```python
from build123d import *

# Parameters (mm, degrees)
F0_R     = 1.5
F1_DEPTH = 50
F2_R     = 12
F3_R     = 5
F5_DEPTH = 4
F6_SIZE  = 2.5


with BuildPart() as f1:
    # F0 (on Top) → F1 (new body)
    with BuildSketch(Plane.XY):
        with BuildLine():
            Line((40.1261364576, -50), (50, -50))
            Line((50, -50), (50, -40.1261364576))
            ThreePointArc((50, -40.1261364576), (48.5323223277, -39.658202653), (47, -39.5))
            Line((47, -39.5), (47, -47))
            Line((47, -47), (39.5, -47))
            ThreePointArc((39.5, -47), (39.658202653, -48.5323223277), (40.1261364576, -50))
        make_face()
        with BuildLine():
            Line((-40.1261364576, -50), (40.1261364576, -50))
            ThreePointArc((40.1261364576, -50), (39.658202653, -48.5323223277), (39.5, -47))
            Line((39.5, -47), (-39.5, -47))
            ThreePointArc((-39.5, -47), (-39.658202653, -48.5323223277), (-40.1261364576, -50))
        make_face()
        with BuildLine():
            ThreePointArc((47, -39.5), (48.5323223277, -39.658202653), (50, -40.1261364576))
            Line((50, -40.1261364576), (50, 40.1261364576))
            ThreePointArc((50, 40.1261364576), (48.5323223277, 39.658202653), (47, 39.5))
            Line((47, 39.5), (47, -39.5))
        make_face()
        with BuildLine():
            Line((-50, -50), (-40.1261364576, -50))
            ThreePointArc((-40.1261364576, -50), (-39.658202653, -48.5323223277), (-39.5, -47))
            Line((-39.5, -47), (-44, -47))
            Line((-44, -47), (-47, -47))
            ThreePointArc((-47, -47), (-50.0530276117, -44.8189291928), (-52.9544285232, -42.4398705103))
            ThreePointArc((-52.9544285232, -42.4398705103), (-53.9803824114, -44.2569612852), (-54.4659740059, -46.2863949669))
            ThreePointArc((-54.4659740059, -46.2863949669), (-52.2760251532, -48.1949550771), (-50, -50))
        make_face()
        with BuildLine():
            ThreePointArc((47, -39.5), (41.6966991411, -41.6966991411), (39.5, -47))
            Line((39.5, -47), (47, -47))
            Line((47, -47), (47, -39.5))
        make_face()
        with Locations((44, -44)):
            Circle(F0_R, mode=Mode.SUBTRACT)
        with BuildLine():
            ThreePointArc((47, 39.5), (48.5323223277, 39.658202653), (50, 40.1261364576))
            Line((50, 40.1261364576), (50, 50))
            Line((50, 50), (40.1261364576, 50))
            ThreePointArc((40.1261364576, 50), (39.658202653, 48.5323223277), (39.5, 47))
            Line((39.5, 47), (44, 47))
            Line((44, 47), (47, 47))
            Line((47, 47), (47, 44))
            Line((47, 44), (47, 39.5))
        make_face()
        with BuildLine():
            ThreePointArc((-54.4659740059, 46.2863949669), (-74.8805891399, 0), (-54.4659740059, -46.2863949669))
            ThreePointArc((-54.4659740059, -46.2863949669), (-53.9803824114, -44.2569612852), (-52.9544285232, -42.4398705103))
            ThreePointArc((-52.9544285232, -42.4398705103), (-67.1504896249, -23.2960258249), (-72.1814061329, 0))
            ThreePointArc((-72.1814061329, 0), (-67.1504896249, 23.2960258249), (-52.9544285232, 42.4398705103))
            ThreePointArc((-52.9544285232, 42.4398705103), (-53.9803824114, 44.2569612852), (-54.4659740059, 46.2863949669))
        make_face()
        with BuildLine():
            Line((-44, -47), (-39.5, -47))
            ThreePointArc((-39.5, -47), (-44.5925338968, -39.8968945551), (-52.9544285232, -42.4398705103))
            ThreePointArc((-52.9544285232, -42.4398705103), (-50.0530276117, -44.8189291928), (-47, -47))
            Line((-47, -47), (-44, -47))
        make_face()
        with BuildLine():
            ThreePointArc((-42.5, -44), (-42.9393398282, -45.0606601718), (-44, -45.5))
            ThreePointArc((-44, -45.5), (-45.0606601718, -45.0606601718), (-45.5, -44))
            ThreePointArc((-45.5, -44), (-44, -42.5), (-42.5, -44))
        make_face(mode=Mode.SUBTRACT)
        with BuildLine():
            ThreePointArc((39.5, 47), (41.6966991411, 41.6966991411), (47, 39.5))
            Line((47, 39.5), (47, 44))
            Line((47, 44), (45.5, 44))
            ThreePointArc((45.5, 44), (42.9393398282, 42.9393398282), (44, 45.5))
            Line((44, 45.5), (44, 47))
            Line((44, 47), (39.5, 47))
        make_face()
        with BuildLine():
            ThreePointArc((-50, 50), (-52.2760251532, 48.1949550771), (-54.4659740059, 46.2863949669))
            ThreePointArc((-54.4659740059, 46.2863949669), (-53.9803824114, 44.2569612852), (-52.9544285232, 42.4398705103))
            ThreePointArc((-52.9544285232, 42.4398705103), (-50.0530276117, 44.8189291928), (-47, 47))
            Line((-47, 47), (-39.5, 47))
            ThreePointArc((-39.5, 47), (-39.658202653, 48.5323223277), (-40.1261364576, 50))
            Line((-40.1261364576, 50), (-50, 50))
        make_face()
        with BuildLine():
            ThreePointArc((39.5, 47), (39.658202653, 48.5323223277), (40.1261364576, 50))
            Line((40.1261364576, 50), (-40.1261364576, 50))
            ThreePointArc((-40.1261364576, 50), (-39.658202653, 48.5323223277), (-39.5, 47))
            Line((-39.5, 47), (39.5, 47))
        make_face()
        with BuildLine():
            Line((45.5, 44), (47, 44))
            Line((47, 44), (47, 47))
            Line((47, 47), (44, 47))
            Line((44, 47), (44, 45.5))
            ThreePointArc((44, 45.5), (45.0606601718, 45.0606601718), (45.5, 44))
        make_face()
        with BuildLine():
            ThreePointArc((-47, 47), (-50.0530276117, 44.8189291928), (-52.9544285232, 42.4398705103))
            ThreePointArc((-52.9544285232, 42.4398705103), (-44.5925338968, 39.8968945551), (-39.5, 47))
            Line((-39.5, 47), (-47, 47))
        make_face()
        with Locations((-44, 44)):
            Circle(F0_R, mode=Mode.SUBTRACT)
    extrude(amount=F1_DEPTH)

    # F2
    f2_edges = [f1.edges().sort_by_distance(p)[0] for p in [
        (-50, 50, 25),
        (50, 50, 25),
        (50, -50, 25),
        (-50, -50, 25),
    ]]
    fillet(f2_edges, radius=F2_R)

    # F3
    f3_edges = [f1.edges().sort_by_distance(p)[0] for p in [
        (-39.5, -47, 25),
        (39.5, -47, 25),
        (47, -39.5, 25),
        (39.5, 47, 25),
        (47, 39.5, 25),
        (-39.5, 47, 25),
        (-52.954429, -42.439871, 25),
        (-52.954429, 42.439871, 25),
    ]]
    fillet(f3_edges, radius=F3_R)

    # F4 (on face) → F5 (cut)
    with BuildSketch(Plane.YZ.offset(50)):
        with BuildLine():
            Line((-22.25, 8.4361030432), (-22.25, 27.5638969568))
            ThreePointArc((-22.25, 27.5638969568), (-29.825, 18), (-22.25, 8.4361030432))
        make_face()
        with BuildLine():
            Line((-17.75, 8.4361030432), (-17.75, 27.5638969568))
            ThreePointArc((-17.75, 27.5638969568), (-20, 27.825), (-22.25, 27.5638969568))
            Line((-22.25, 27.5638969568), (-22.25, 8.4361030432))
            ThreePointArc((-22.25, 8.4361030432), (-20, 8.175), (-17.75, 8.4361030432))
        make_face()
        with BuildLine():
            ThreePointArc((-17.75, 8.4361030432), (-12.2981536305, 11.8998206994), (-10.175, 18))
            ThreePointArc((-10.175, 18), (-12.2981536305, 24.1001793006), (-17.75, 27.5638969568))
            Line((-17.75, 27.5638969568), (-17.75, 8.4361030432))
        make_face()
        with BuildLine():
            ThreePointArc((-22.25, 27.5638969568), (-20, 27.825), (-17.75, 27.5638969568))
            Line((-17.75, 27.5638969568), (-17.75, 29.05))
            Line((-17.75, 29.05), (-22.25, 29.05))
            Line((-22.25, 29.05), (-22.25, 27.5638969568))
        make_face()
        with BuildLine():
            Line((-17.75, 6.95), (-17.75, 8.4361030432))
            ThreePointArc((-17.75, 8.4361030432), (-20, 8.175), (-22.25, 8.4361030432))
            Line((-22.25, 8.4361030432), (-22.25, 6.95))
            Line((-22.25, 6.95), (-17.75, 6.95))
        make_face()
    extrude(amount=-F5_DEPTH, mode=Mode.SUBTRACT)

    # F6
    f6_edges = [f1.edges().sort_by_distance(p)[0] for p in [
        (47, -20, 29.05),
        (47, -20, 6.95),
    ]]
    chamfer(f6_edges, length=F6_SIZE)


solid = f1.part
```
Part model, mm, in its own coordinate system. A direction names the side the tool comes from. Round coordinates to 2 decimals unless told otherwise and drop trailing zeros. Order: outer loops, then holes, each group sorted by start corner. A loop starts at its lowest first (then second) coordinate and runs counter-clockwise, first axis right, second up. Notation, with made-up numbers: M 39,73 L 96,73 A5 cw 96,81 Z; hole C 33,31.5 d7. An arc over 180 degrees is marked long. Answer in a Markdown table with one row per item. Add a question column.
Q1. Cut at B-B on y = 17. Give the cut face in (x, z).
Q2. Wall check: L1, parallel to Y at x = -44, z = 40; L2, parallel to Y at x = 17.5, z = 14; L3, parallel to Y at x = 44, z = 27. Give the ranges that are in metal, low to high. Write a range as from..to.
Q3. Cut at A-A on x = -20. Give the cut face in (y, z), and give its area (3 significant figures).
Q4. Cut at C-C on z = 13.5. Give the number of separate pieces and of enclosed holes in the cut face, and give its area (3 significant figures).
Q5. Mould opens along Z. For faces 4 (the face through (-8, 48, 50)), 5 (the face through (48, -17.75, 7)), 6 (the face through (48, -22.25, 7)), 7 (the face through (0, 47, 25)) say: +Z half, -Z half, draft (parallel to the pull), parting line (faces both ways), or undercut.
Q6. 3-axis set-ups, long thin cutter, end or side, ignore diameter. For faces 1 (the face through (-49.921, 49.246, 25.35)), 2 (the face through (38.32, -46.16, 25.35)), 3 (the face through (48.521, -29.823, 18.184)): which of +Z, -Z, +X, -X, +Y, -Y reach the whole face in a straight line?
Q7. Pin check, flat tips, straight feed: pin 1 (1.5 mm diameter, centred on y = 30, z = 19, fed in from -X); pin 2 (3.5 mm diameter, centred on x = 48.5, z = 29.5, fed in from -Y); pin 3 (2 mm diameter, centred on y = 4, z = 11, fed in from -X). Stop position of each tip, or through.
Established:
| question | item | result |
|---|---|---|
| 1 | outline | M -72.53,0 L -69.56,0 L -69.56,50 L -72.53,50 Z; M 47,0 L 50,0 L 50,50 L 47,50 Z |
| 2 | L1 | y = -50..-45.5, -42.5..-40.13, 40.13..42.5, 45.5..50 |
| 2 | L2 | y = -50..-47, 47..50 |
| 2 | L3 | y = -48.39..-45.5, -42.5..-40.13, 40.13..42.5, 45.5..48.39 |
| 3 | outline | M -50,0 L -47,0 L -47,50 L -50,50 Z; M 47,0 L 50,0 L 50,50 L 47,50 Z |
| 3 | area | 300 mm2 |
| 4 | separate pieces | 1 |
| 4 | enclosed holes | 4 |
| 4 | area | 1,340 mm2 |
| 5 | face 4 | +Z half |
| 5 | face 5 | undercut |
| 5 | face 6 | undercut |
| 5 | face 7 | draft |
| 6 | face 1 | +Z, -Z, -X, +Y |
| 6 | face 2 | +Z, -Z |
| 6 | face 3 | +X |
| 7 | pin 1 | stops at x = -67.64 |
| 7 | pin 2 | stops at y = -46.21 |
| 7 | pin 3 | stops at x = -74.81 |
